Source: CAD feature listing. Evaluate the final solid. Frame: model axes, mm. Give positions to 0.01 mm unless a question says otherwise; leave off trailing zeros. Order: outer loops, then holes, each group sorted by start corner. A loop starts at its lowest first (then second) coordinate and runs counter-clockwise, first axis right, second up. Notation, with made-up numbers: M -23,34 L 7,34 A16 ccw 7,55 Z; hole C 18,-4.5 d5. An arc over 180 degrees is marked long. Return JSON: item names as keys, results as strings.
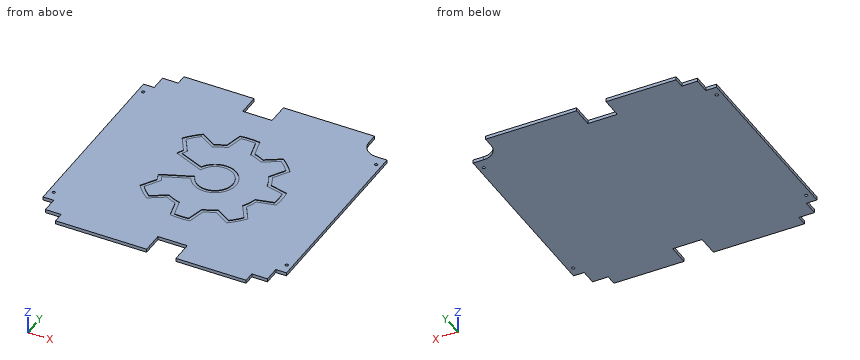
from build123d import *

# Parameters (mm, degrees)
SKETCH1_R           = 2.75
BOSS_EXTRUDE1_DEPTH = 6.35
CUT_EXTRUDE1_DEPTH  = 6.35
CUT_EXTRUDE2_DEPTH  = 1


with BuildPart() as part:
    # Sketch1 → Boss-Extrude1 (new body)
    with BuildSketch(Plane.XY):
        Polygon((182, -212), (212, -212), (212, -182), (232.5, -182), (232.5, 0), (232.5, 182), (212, 182), (212, 212), (182, 212), (182, 232.5), (8, 232.5), (8, 191.5), (-48, 191.5), (-48, 232.5), (-182, 232.5), (-182, 212), (-212, 212), (-212, 182), (-232.5, 182), (-232.5, 0), (-232.5, -182), (-212, -182), (-212, -212), (-182, -212), (-182, -232.5), (-8, -232.5), (-8, -191.5), (48, -191.5), (48, -232.5), (182, -232.5), align=None)
        with Locations((-222.5, -162)):
            Circle(SKETCH1_R, mode=Mode.SUBTRACT)
        with Locations((222.5, -162)):
            Circle(SKETCH1_R, mode=Mode.SUBTRACT)
        with Locations((222.5, 162)):
            Circle(SKETCH1_R, mode=Mode.SUBTRACT)
        with Locations((-222.5, 162)):
            Circle(SKETCH1_R, mode=Mode.SUBTRACT)
    extrude(amount=BOSS_EXTRUDE1_DEPTH)

    # Sketch2 → Cut-Extrude1 (cut)
    with BuildSketch(Plane.XY.offset(6.35)):
        with BuildLine():
            Line((212, 212), (182, 212))
            ThreePointArc((182, 212), (190.786796564, 190.786796564), (212, 182))
            Line((212, 182), (212, 212))
        make_face()
    extrude(amount=-CUT_EXTRUDE1_DEPTH, mode=Mode.SUBTRACT)

    # Sketch3 → Cut-Extrude2 (cut)
    with BuildSketch(Plane.XY.offset(6.35)):
        with BuildLine():
            Line((-90.71398693, 34.138368447), (-32.791230158, 10.145977022))
            ThreePointArc((-32.791230158, 10.145977022), (34.325, 0), (-32.791230158, -10.145977022))
            Line((-32.791230158, -10.145977022), (-90.71398693, -34.138368447))
            ThreePointArc((-90.71398693, -34.138368447), (-88.022539954, -40.576940312), (-84.874800654, -46.805168935))
            Line((-84.874800654, -46.805168935), (-103.008511577, -76.276321146))
            ThreePointArc((-103.008511577, -76.276321146), (-90.633411679, -90.633411679), (-76.276321146, -103.008511577))
            Line((-76.276321146, -103.008511577), (-46.805168935, -84.874800654))
            ThreePointArc((-46.805168935, -84.874800654), (-37.091591682, -89.547023689), (-26.919294746, -93.111799442))
            Line((-26.919294746, -93.111799442), (-18.90251313, -126.773520983))
            ThreePointArc((-18.90251313, -126.773520983), (0, -128.175), (18.90251313, -126.773520983))
            Line((18.90251313, -126.773520983), (26.919294746, -93.111799442))
            ThreePointArc((26.919294746, -93.111799442), (37.091591682, -89.547023689), (46.805168935, -84.874800654))
            Line((46.805168935, -84.874800654), (76.276321146, -103.008511577))
            ThreePointArc((76.276321146, -103.008511577), (90.633411679, -90.633411679), (103.008511577, -76.276321146))
            Line((103.008511577, -76.276321146), (84.874800654, -46.805168935))
            ThreePointArc((84.874800654, -46.805168935), (89.547023689, -37.091591682), (93.111799442, -26.919294746))
            Line((93.111799442, -26.919294746), (126.773520983, -18.90251313))
            ThreePointArc((126.773520983, -18.90251313), (128.175, 0), (126.773520983, 18.90251313))
            Line((126.773520983, 18.90251313), (93.111799442, 26.919294746))
            ThreePointArc((93.111799442, 26.919294746), (89.547023689, 37.091591682), (84.874800654, 46.805168935))
            Line((84.874800654, 46.805168935), (103.008511577, 76.276321146))
            ThreePointArc((103.008511577, 76.276321146), (90.633411679, 90.633411679), (76.276321146, 103.008511577))
            Line((76.276321146, 103.008511577), (46.805168935, 84.874800654))
            ThreePointArc((46.805168935, 84.874800654), (37.091591682, 89.547023689), (26.919294746, 93.111799442))
            Line((26.919294746, 93.111799442), (18.90251313, 126.773520983))
            ThreePointArc((18.90251313, 126.773520983), (0, 128.175), (-18.90251313, 126.773520983))
            Line((-18.90251313, 126.773520983), (-26.919294746, 93.111799442))
            ThreePointArc((-26.919294746, 93.111799442), (-37.091591682, 89.547023689), (-46.805168935, 84.874800654))
            Line((-46.805168935, 84.874800654), (-76.276321146, 103.008511577))
            ThreePointArc((-76.276321146, 103.008511577), (-90.633411679, 90.633411679), (-103.008511577, 76.276321146))
            Line((-103.008511577, 76.276321146), (-84.874800654, 46.805168935))
            ThreePointArc((-84.874800654, 46.805168935), (-88.022539954, 40.576940312), (-90.71398693, 34.138368447))
        make_face()
        with BuildLine():
            Line((-82.41394096, 37.57356731), (-36.249121046, 18.451472797))
            ThreePointArc((-36.249121046, 18.451472797), (40.675, 0), (-36.249121046, -18.451472797))
            Line((-36.249121046, -18.451472797), (-82.41394096, -37.57356731))
            ThreePointArc((-82.41394096, -37.57356731), (-80.084171036, -42.312600659), (-77.482180911, -46.907806027))
            Line((-77.482180911, -46.907806027), (-95.308362806, -75.879157904))
            ThreePointArc((-95.308362806, -75.879157904), (-86.143283618, -86.143283618), (-75.879157904, -95.308362806))
            Line((-75.879157904, -95.308362806), (-46.907806027, -77.482180911))
            ThreePointArc((-46.907806027, -77.482180911), (-34.661551886, -83.680388657), (-21.619347811, -87.957003276))
            Line((-21.619347811, -87.957003276), (-13.73852254, -121.047856749))
            ThreePointArc((-13.73852254, -121.047856749), (0, -121.825), (13.73852254, -121.047856749))
            Line((13.73852254, -121.047856749), (21.619347811, -87.957003276))
            ThreePointArc((21.619347811, -87.957003276), (34.661551886, -83.680388657), (46.907806027, -77.482180911))
            Line((46.907806027, -77.482180911), (75.879157904, -95.308362806))
            ThreePointArc((75.879157904, -95.308362806), (86.143283618, -86.143283618), (95.308362806, -75.879157904))
            Line((95.308362806, -75.879157904), (77.482180911, -46.907806027))
            ThreePointArc((77.482180911, -46.907806027), (83.680388657, -34.661551886), (87.957003276, -21.619347811))
            Line((87.957003276, -21.619347811), (121.047856749, -13.73852254))
            ThreePointArc((121.047856749, -13.73852254), (121.825, 0), (121.047856749, 13.73852254))
            Line((121.047856749, 13.73852254), (87.957003276, 21.619347811))
            ThreePointArc((87.957003276, 21.619347811), (83.680388657, 34.661551886), (77.482180911, 46.907806027))
            Line((77.482180911, 46.907806027), (95.308362806, 75.879157904))
            ThreePointArc((95.308362806, 75.879157904), (86.143283618, 86.143283618), (75.879157904, 95.308362806))
            Line((75.879157904, 95.308362806), (46.907806027, 77.482180911))
            ThreePointArc((46.907806027, 77.482180911), (34.661551886, 83.680388657), (21.619347811, 87.957003276))
            Line((21.619347811, 87.957003276), (13.73852254, 121.047856749))
            ThreePointArc((13.73852254, 121.047856749), (0, 121.825), (-13.73852254, 121.047856749))
            Line((-13.73852254, 121.047856749), (-21.619347811, 87.957003276))
            ThreePointArc((-21.619347811, 87.957003276), (-34.661551886, 83.680388657), (-46.907806027, 77.482180911))
            Line((-46.907806027, 77.482180911), (-75.879157904, 95.308362806))
            ThreePointArc((-75.879157904, 95.308362806), (-86.143283618, 86.143283618), (-95.308362806, 75.879157904))
            Line((-95.308362806, 75.879157904), (-77.482180911, 46.907806027))
            ThreePointArc((-77.482180911, 46.907806027), (-80.084171036, 42.312600659), (-82.41394096, 37.57356731))
        make_face(mode=Mode.SUBTRACT)
    extrude(amount=-CUT_EXTRUDE2_DEPTH, mode=Mode.SUBTRACT)


solid = part.part
1. First-contact query: pin 1 (3 mm diameter, centred on y = 224, z = 4.5, fed in from +X); pin 2 (1 mm diameter, centred on x = -88, y = 85.5, fed in from +Z); pin 3 (1.9 mm diameter, centred on x = -220.5, z = 2.5, fed in from +Y). Flat tips, straight axial feed; report the tip coordinate or a pass-through.
Evaluation:
{"pin 1": "stops at x = 182", "pin 2": "stops at z = 5.35", "pin 3": "stops at y = 182"}
2. Ray query, probe 1 along X at (y, z) = (-162, 1.75); probe 2 along Y at (x, z) = (-222.5, 2.75); probe 3 along X at (y, z) = (66, 5.75). Return the intervals inside material, ascending.
Evaluation:
{"probe 1": "x = -232.5 to -225.25, -219.75 to 219.75, 225.25 to 232.5", "probe 2": "y = -182 to -164.75, -159.25 to 159.25, 164.75 to 182", "probe 3": "x = -232.5 to -96.69, -89.23 to 89.23, 96.69 to 232.5"}
3. Section query A-A (z = 3). State how many separate pieces and enclosed holes the cut face has, then the cut area to 3 significant figures.
Evaluation:
{"separate pieces": "1", "enclosed holes": "4", "area": "204,000 mm^2"}
4. Section query B-B (x = -2.5). Return loops of the section in (y, z).
Evaluation:
{"outline": "M -191.5,0 L 191.5,0 L 191.5,6.35 L 128.15,6.35 L 128.15,5.35 L 121.8,5.35 L 121.8,6.35 L 40.6,6.35 L 40.6,5.35 L 34.23,5.35 L 34.23,6.35 L -34.23,6.35 L -34.23,5.35 L -40.6,5.35 L -40.6,6.35 L -121.8,6.35 L -121.8,5.35 L -128.15,5.35 L -128.15,6.35 L -191.5,6.35 Z"}
